The figure shows three views and two pictorial views of one solid part (mm, origin at its lowest corner). Answer the questions. A direction names the side the tool comes from. Give positions to 0.01 mm unless a question says otherwise; leave off trailing zeros. Order: outer loops, then holes, each group sorted by start corner. A loop starts at its lowest first (then second) coordinate and runs counter-clockwise, first axis right, second up. Notation, with made-up numbers: (51.5, 13) - (79.5, 13) arc R16 cw to (79.5, 32) - close; hole circle Ø6 at (45.25, 33.25). An arc over 180 degrees is marked (long way). Answer as CSV lines item,"result". Start each with the question number.
1. Section B-B on z = 2.5 is taken. Give the vertices of the cut face in (x, y).
2. Consider line 1 along Z through (x, y) = (4, 2.8); line 2 along X through (y, z) = (3, 3); line 3 along X through (y, z) = (1.3, 1.75) (1 decimal). Determine where each line is inside the solid, lowest interval first. Write a range as [from, to].
3. Which of the six approach directions +Z, -Z, +X, -X, +Y, -Y give full straight-line access (tool end or side, diameter ignored) to the marked faces 5 and 6?
4. Determine the mould class of the marked faces 1, 2, 3 and 4 for opening direction X: +X half, -X half, draft (parallel to the pull), parting line (faces both ways), or undercut.
5. Section A-A on x = 3.5 is taken. Give the vertices of the cut face in (y, z), and give its area (3 significant figures).
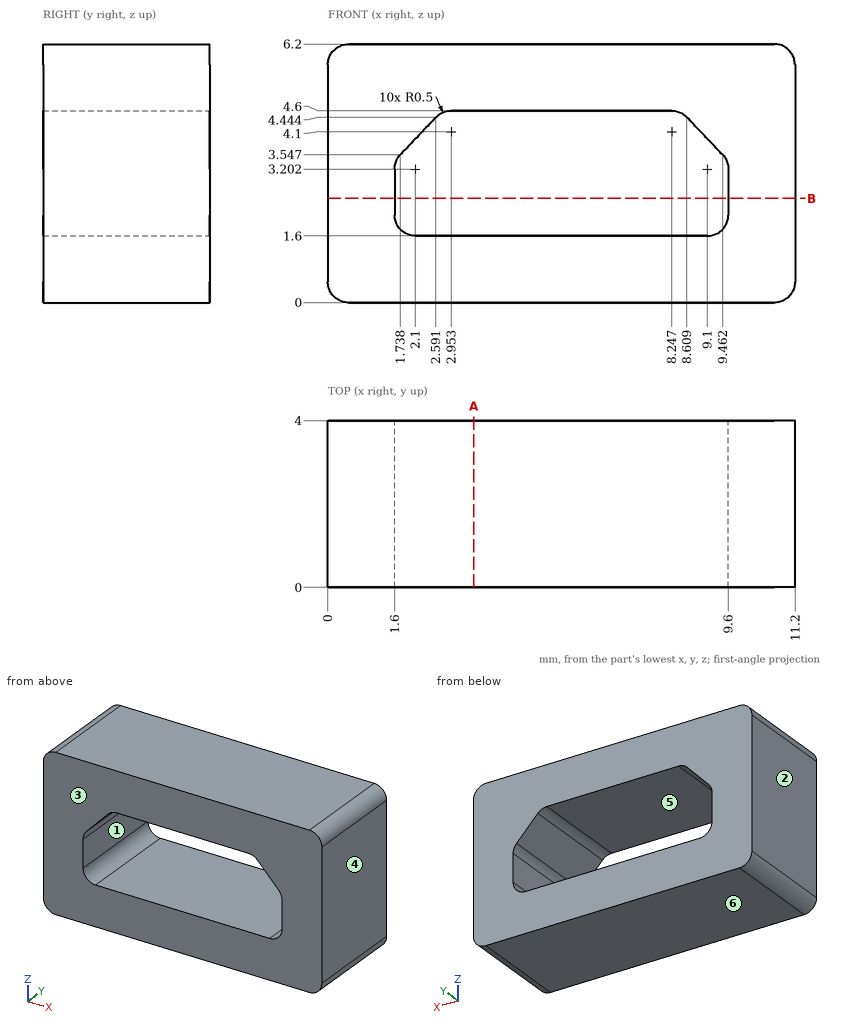
Checks:
1,outline,"(0, 0) - (1.6, 0) - (1.6, 4) - (0, 4) - close; (9.6, 0) - (11.2, 0) - (11.2, 4) - (9.6, 4) - close"
2,line 1,"z = [0, 1.6], [4.6, 6.2]"
2,line 2,"x = [0, 1.6], [9.6, 11.2]"
2,line 3,"x = [0, 1.7], [9.5, 11.2]"
3,face 5,"+Y, -Y"
3,face 6,"-Z, +X, -X, +Y, -Y"
4,face 1,"undercut"
4,face 2,"-X half"
4,face 3,"draft"
4,face 4,"+X half"
5,outline,"(0, 0) - (4, 0) - (4, 1.6) - (0, 1.6) - close; (0, 4.6) - (4, 4.6) - (4, 6.2) - (0, 6.2) - close"
5,area,"12.8 mm²"
